Verification items for the finished model (mm, model axes). Face numbers are marked on the shaded views. Round coordinates to 2 decimals unless told otherwise and drop trailing zeros. Order: outer loops, then holes, each group sorted by start corner. A loop starts at its lowest first (then second) coordinate and runs counter-clockwise, first axis right, second up. Notation, with made-up numbers: (-30.75, 4.5) -> (-3.75, 4.5) arc R22 cw to (-3.75, 32.5) -> close; hole circle Ø9 at (-33.5, 11.25). An arc over 180 degrees is marked (long way). Return JSON: item names as keys, results as strings. Group by question number.
1) Depth check by flat-ended pin: pin 1 (0.5 mm diameter, centred on x = 1, y = 3, fed in from +Z); pin 2 (3 mm diameter, centred on x = -0.5, z = 0.5, fed in from +Y); pin 3 (1.1 mm diameter, centred on x = -0.5, y = 3, fed in from -Z). Enter the tip coordinate at first touch or a pass-through.
2) Draft check along Z on the marked faces 1, 2 and 3. Enter one of: pulls with the +Z half, pulls with the -Z half, needs draft (parallel to the pull), parting line crosses it, or undercut.
3) Scan lines: L1, parallel to X at y = 2.85, z = 2.5; L2, parallel to X at y = 3.15, z = 0; L3, parallel to X at y = 1.65, z = -2. Record each from-to range of solid material in increasing order.
4) Section check D-D on y = 2.95. Enter the section's corners in (x, z).
5) Section check B-B on x = 0. Enter the section's corners in (y, z), plus the area to 3 significant figures.
6) Section check A-A on y = 0.85. Enter the section's corners in (x, z), plus the area to 3 significant figures.
7) Section check C-C on x = 6. Enter the section's corners in (y, z), plus the area to 3 significant figures.
```python
from build123d import *

# Parameters (mm, degrees)
SKETCH1_R           = 4.08
BOSS_EXTRUDE1_DEPTH = 3.45
SKETCH2_R           = 1.6
CUT_EXTRUDE1_DEPTH  = 3.45
CUT_EXTRUDE2_DEPTH  = 1
SKETCH4_R           = 5.08
CUT_EXTRUDE3_DEPTH  = 2.05
FILLET1_R           = 2


with BuildPart() as part:
    # Sketch1 → Boss-Extrude1 (new body)
    with BuildSketch(Plane(origin=(0, 0, 0), x_dir=(1, 0, 0), z_dir=(0, 1, 0))):
        with BuildLine():
            Line((-15, 7), (15, 7))
            ThreePointArc((15, 7), (22, 0), (15, -7))
            Line((15, -7), (-15, -7))
            ThreePointArc((-15, -7), (-22, 0), (-15, 7))
        make_face()
        with Locations((-15, 0)):
            Circle(SKETCH1_R, mode=Mode.SUBTRACT)
        with Locations((15, 0)):
            Circle(SKETCH1_R, mode=Mode.SUBTRACT)
    extrude(amount=BOSS_EXTRUDE1_DEPTH)

    # Sketch2 → Cut-Extrude1 (cut)
    with BuildSketch(Plane(origin=(0, 3.45, 0), x_dir=(1, 0, 0), z_dir=(0, 1, 0))):
        Circle(SKETCH2_R)
    extrude(amount=-CUT_EXTRUDE1_DEPTH, mode=Mode.SUBTRACT)

    # Sketch3 → Cut-Extrude2 (cut)
    with BuildSketch(Plane(origin=(0, 3.45, 0), x_dir=(1, 0, 0), z_dir=(0, 1, 0))):
        Polygon((-1.645448267, 2.85), (1.645448267, 2.85), (3.290896534, 0), (1.645448267, -2.85), (-1.645448267, -2.85), (-3.290896534, 0), align=None)
    extrude(amount=-CUT_EXTRUDE2_DEPTH, mode=Mode.SUBTRACT)

    # Sketch4 → Cut-Extrude3 (cut)
    with BuildSketch(Plane.XZ):
        with Locations((-15, 0)):
            Circle(SKETCH4_R)
        with Locations((15, 0)):
            Circle(SKETCH4_R)
    extrude(amount=-CUT_EXTRUDE3_DEPTH, mode=Mode.SUBTRACT)

    # Fillet1
    fillet1_edges = [part.edges().sort_by_distance(p)[0] for p in [
        (22, 3.45, 0),
        (0, 3.45, -7),
        (-22, 3.45, 0),
        (0, 3.45, 7),
    ]]
    fillet(fillet1_edges, radius=FILLET1_R)


solid = part.part
```
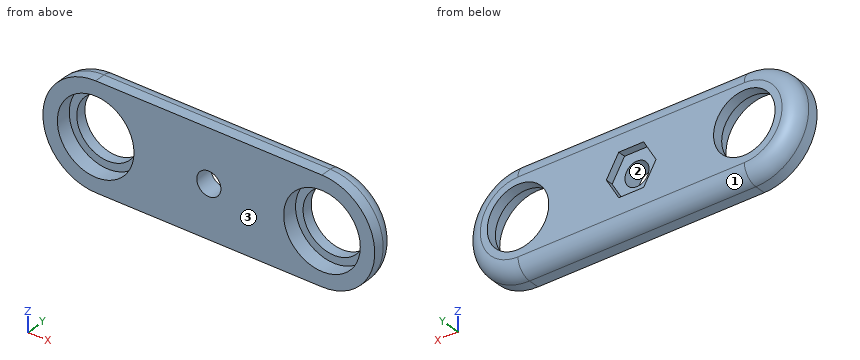
Check result:
{
 "1": {"pin 1": "z = 6.52", "pin 2": "y = 2.45", "pin 3": "z = -6.73"},
 "2": {"face 1": "pulls with the -Z half", "face 2": "undercut", "face 3": "needs draft"},
 "3": {"L1": "-20.92 to -18.22, -11.78 to -1.85, 1.85 to 11.78, 18.22 to 20.92", "L2": "-21.05 to -19.08, -10.92 to -3.29, 3.29 to 10.92, 19.08 to 21.05", "L3": "-21.7 to -19.67, -10.33 to 10.33, 19.67 to 21.7"},
 "4": {"outline": "(-15, -6.32) -> (15, -6.32) arc R6.32 ccw to (15, 6.32) -> (-15, 6.32) arc R6.32 ccw to start; hole circle Ø8.16 at (-15, 0); hole (-3.29, 0) -> (-1.65, -2.85) -> (1.65, -2.85) -> (3.29, 0) -> (1.65, 2.85) -> (-1.65, 2.85) -> close; hole circle Ø8.16 at (15, 0)"},
 "5": {"outline": "(0, -7) -> (1.45, -7) arc R2 ccw to (3.45, -5) -> (3.45, -2.85) -> (2.45, -2.85) -> (2.45, -1.6) -> (0, -1.6) -> close; (0, 1.6) -> (2.45, 1.6) -> (2.45, 2.85) -> (3.45, 2.85) -> (3.45, 5) arc R2 ccw to (1.45, 7) -> (0, 7) -> close", "area": "33.0 mm^2"},
 "6": {"outline": "(-15, -7) -> (15, -7) arc R7 ccw to (15, 7) -> (-15, 7) arc R7 ccw to start; hole circle Ø10.16 at (-15, 0); hole circle Ø3.2 at (0, 0); hole circle Ø10.16 at (15, 0)", "area": "404 mm^2"},
 "7": {"outline": "(0, -7) -> (1.45, -7) arc R2 ccw to (3.45, -5) -> (3.45, 5) arc R2 ccw to (1.45, 7) -> (0, 7) -> close", "area": "46.6 mm^2"}
}
